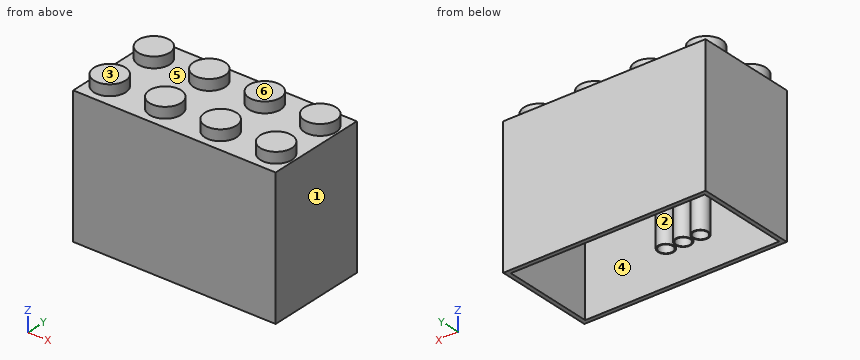
from build123d import *

# Parameters (mm, degrees)
F0_W     = 96
F0_H     = 48
F1_DEPTH = 65
F2_R     = 7.5
F3_DEPTH = 5.1
F4_T     = -2
F5_R     = 3.75
F5_R_2   = 3.25
F6_DEPTH = 63
F8_DEPTH = 6.5


# Not quite as in the source:
# - after a boolean that leaves OpenCascade's solid faulty, fix() repairs it


with BuildPart() as f1:
    # F0 (on Top) → F1 (new body)
    with BuildSketch(Plane.XY):
        Rectangle(F0_W, F0_H)
    extrude(amount=F1_DEPTH)

    # F2 (on face) → F3 (join)
    with BuildSketch(Plane.XY.offset(65)):
        with Locations((-39.45, 13.05)):
            Circle(F2_R)
        with Locations((-13.15, 13.05)):
            Circle(F2_R)
        with Locations((39.45, 13.05)):
            Circle(F2_R)
        with Locations((39.45, -13.05)):
            Circle(F2_R)
        with Locations((13.15, -13.05)):
            Circle(F2_R)
        with Locations((-13.15, -13.05)):
            Circle(F2_R)
        with Locations((-39.45, -13.05)):
            Circle(F2_R)
        with Locations((13.15, 13.05)):
            Circle(F2_R)
    extrude(amount=F3_DEPTH)

    # F4
    f4_openings = [f1.faces().sort_by_distance(p)[0] for p in [
        (0, 0, 0),
    ]]
    offset(amount=F4_T, openings=f4_openings, kind=Kind.INTERSECTION)

    # F5 (on face) → F6 (join, through all)
    with BuildSketch(Plane(origin=(0, 0, 63), x_dir=(1, 0, 0), z_dir=(0, 0, -1))):
        with Locations((-26.3, 0)):
            Circle(F5_R)
        with Locations((-26.3, 0)):
            Circle(F5_R_2, mode=Mode.SUBTRACT)
        with Locations((-18.1, 0)):
            Circle(F5_R)
        with Locations((-18.1, 0)):
            Circle(F5_R_2, mode=Mode.SUBTRACT)
        with Locations((-9.9, 0)):
            Circle(F5_R)
        with Locations((-9.9, 0)):
            Circle(F5_R_2, mode=Mode.SUBTRACT)
    extrude(amount=F6_DEPTH)

    # F7 (on face) → F8 (join)
    with BuildSketch(Plane(origin=(0, 0, 63), x_dir=(1, 0, 0), z_dir=(0, 0, -1))):
        with BuildLine():
            ThreePointArc((-20.1, 3.1721443851), (-18.1, 3.75), (-16.1, 3.1721443851))
            Line((-16.1, 3.1721443851), (-16.1, 8.4080715214))
            ThreePointArc((-16.1, 8.4080715214), (-18.65, 13.05), (-16.1, 17.6919284786))
            Line((-16.1, 17.6919284786), (-16.1, 22))
            Line((-16.1, 22), (-20.1, 22))
            Line((-20.1, 22), (-20.1, 3.1721443851))
        make_face()
        with BuildLine():
            Line((-16.1, -8.4080715214), (-16.1, -3.1721443851))
            ThreePointArc((-16.1, -3.1721443851), (-18.1, -3.75), (-20.1, -3.1721443851))
            Line((-20.1, -3.1721443851), (-20.1, -22))
            Line((-20.1, -22), (-16.1, -22))
            Line((-16.1, -22), (-16.1, -17.6919284786))
            ThreePointArc((-16.1, -17.6919284786), (-18.65, -13.05), (-16.1, -8.4080715214))
        make_face()
    extrude(amount=F8_DEPTH)

    add(f1.part.fix(), mode=Mode.REPLACE)


solid = f1.part
Read the model definition and answer for the solid it produces. Units are mm, in the model's axes. Face numbers are marked on the shaded views. A direction names the side the tool comes from. Round coordinates to 2 decimals unless told otherwise and drop trailing zeros. Write each loop counter-clockwise with the first axis right and the second up, starting at its lowest first coordinate (ties: lowest second). Pieces come first, ordered by that corner, then holes. Notation, with made-up numbers: (-36.5, 63.5) - (13.5, 63.5) arc R11 ccw to (13.5, 67.5) - close; hole circle Ø9 at (66.25, 27). An arc over 180 degrees is marked (long way). One line per question, with ' | ' between items. Start each with the question number.
1. Section A-A (z = 52.5) is taken. Determine the outline of the cut face in (x, y).
2. Section C-C (x = -39.45) is taken. Determine the outline of the cut face in (y, z).
3. Section B-B (x = -4.5) is taken. Determine the outline of the cut face in (y, z).
4. Find the intervals of material crossed by probe 1 along X at (y, z) = (13, 64); probe 2 along Y at (x, z) = (-13.15, 66.1); probe 3 along Y at (x, z) = (-34, 37.5), in increasing order. Write a range as [from, to].
5. Each of these flat-tipped pins is pushed along its axis until it touches: pin 1 (12 mm diameter, centred on x = -11, y = 13.5, fed in from -Z); pin 2 (2 mm diameter, centred on x = -17, y = 16, fed in from -Z). Where does it stop, or does it pass through?
6. For the marked faces 4, 5 and 6, determine the directions among +Z, -Z, +X, -X, +Y, -Y from which every point of the face is accessible in a straight line to the end or side of a thin tool.
7. For a pull along X with two mould halves and no side action, classify the marked faces 1, 2 and 3 as +X half, -X half, draft (parallel to the pull), parting line (faces both ways), or undercut.
Filled in:
1) outline: (-48, -24) - (48, -24) - (48, 24) - (-48, 24) - close; circle Ø7.5 at (-26.3, 0); circle Ø7.5 at (-18.1, 0); circle Ø7.5 at (-9.9, 0); hole (-46, -22) - (46, -22) - (46, 22) - (-46, 22) - close; hole circle Ø6.5 at (-26.3, 0); hole circle Ø6.5 at (-18.1, 0); hole circle Ø6.5 at (-9.9, 0)
2) outline: (-24, 0) - (-22, 0) - (-22, 63) - (-18.55, 63) - (-18.55, 68.1) - (-7.55, 68.1) - (-7.55, 63) - (7.55, 63) - (7.55, 68.1) - (18.55, 68.1) - (18.55, 63) - (22, 63) - (22, 0) - (24, 0) - (24, 65) - (20.55, 65) - (20.55, 70.1) - (5.55, 70.1) - (5.55, 65) - (-5.55, 65) - (-5.55, 70.1) - (-20.55, 70.1) - (-20.55, 65) - (-24, 65) - close
3) outline: (-24, 0) - (-22, 0) - (-22, 63) - (22, 63) - (22, 0) - (24, 0) - (24, 65) - (-24, 65) - close
4) probe 1: [-48, -44.95], [-33.95, -18.65], [-7.65, 7.65], [18.65, 33.95], [44.95, 48] | probe 2: [-20.55, -18.55], [-7.55, -5.55], [5.55, 7.55], [18.55, 20.55] | probe 3: [-24, -22], [22, 24]
5) pin 1: z = 63 | pin 2: z = 56.5
6) face 4: -Z | face 5: +Z | face 6: +Z, +X, -X, +Y, -Y
7) face 1: +X half | face 2: undercut | face 3: draft
